Could you check a few things on this model? Use its own coordinates, in mm. Round coordinates to 2 decimals unless told otherwise and drop trailing zeros. Write each loop counter-clockwise with the first axis right and the second up, starting at its lowest first coordinate (ties: lowest second). Pieces come first, ordered by that corner, then holes. Notation, with made-up numbers: M 4,45.5 L 61,45.5 A19 cw 61,59.5 Z; hole C 38.5,-35.5 d1. An arc over 180 degrees is marked long. One line per item, written item: value. Start each with the question number.
(1) I want a section at B-B on y = -10. Please give me the cut outline in (x, z) (3 decimals), and give its area (3 significant figures).
(2) If I drill on L1, parallel to X at y = 7, z = -32 (3 decimals); L2, parallel to Z at x = 297, y = -29 (3 decimals); L3, parallel to X at y = 0, z = 3 (3 decimals), over which ranges is the centre line in solid material (lowest first)?
(3) I'm going to push flat-ended pins straight in: pin 1 Ø4 at (y, z) = (-24.5, 19.5) entering from +X (3 decimals); pin 2 Ø8 at (y, z) = (-5.5, -34) entering from +X (3 decimals); pin 3 Ø5 at (y, z) = (19.5, 1.5) entering from +X (3 decimals). Where does each tip first touch, or does it pass through?
(4) I want a section at A-A on x = 84. Please give me the cut outline in (y, z), and give its area (3 significant figures).
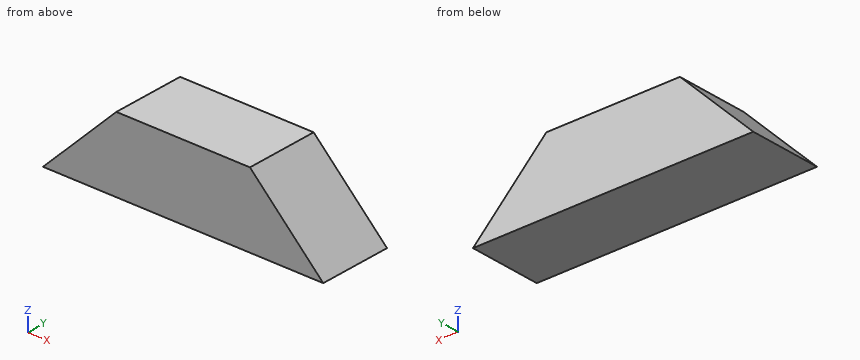
```python
from build123d import *

# Parameters (mm, degrees)
F0_W     = 88.9
F0_H     = 88.9
F1_DEPTH = 339.725
F3_DEPTH = 88.901
F5_DEPTH = 88.901


with BuildPart() as f1:
    # F0 (on Right) → F1 (new body)
    with BuildSketch(Plane.YZ):
        with Locations((1.808545, 0)):
            Rectangle(F0_W, F0_H)
    extrude(amount=F1_DEPTH)

    # F2 (on face) → F3 (cut, through all)
    with BuildSketch(Plane.XZ.offset(42.641455)):
        Polygon((0, 44.45), (0, -44.45), (88.9, 44.45), align=None)
    extrude(amount=-F3_DEPTH, mode=Mode.SUBTRACT)

    # F4 (on face) → F5 (cut, through all)
    with BuildSketch(Plane.XZ.offset(42.641455)):
        Polygon((250.825, 44.45), (339.725, -44.45), (339.725, 44.45), align=None)
    extrude(amount=-F5_DEPTH, mode=Mode.SUBTRACT)


solid = f1.part
```
Found:
1. outline: M 0,-44.45 L 339.725,-44.45 L 250.825,44.45 L 88.9,44.45 Z
1. area: 22,300 mm²
2. L1: x = 12.45 to 327.275
2. L2: z = -44.45 to -1.725
2. L3: x = 47.45 to 292.275
3. pin 1: stops at x = 277.775
3. pin 2: stops at x = 333.275
3. pin 3: stops at x = 296.275
4. outline: M -42.64,-44.45 L 46.26,-44.45 L 46.26,39.55 L -42.64,39.55 Z
4. area: 7,470 mm²
